from build123d import *

# Parameters (mm, degrees)
ESQUISSE2_R             = 7.5
BOSS_EXTRU_1_DEPTH      = 60
ESQUISSE3_R             = 10
BOSS_EXTRU_2_DEPTH      = 15
ESQUISSE4_R             = 10
BOSS_EXTRU_3_DEPTH      = 15
ESQUISSE5_R             = 7.5
BOSS_EXTRU_4_DEPTH      = 14.25
ENL_V_MAT_EXTRU_1_DEPTH = 16


with BuildPart() as part:
    # Esquisse2 → Boss.-Extru.1 (new body)
    with BuildSketch(Plane.XY):
        Circle(ESQUISSE2_R)
    extrude(amount=BOSS_EXTRU_1_DEPTH)

    # Esquisse3 → Boss.-Extru.2 (add)
    with BuildSketch(Plane.XY.offset(60)):
        with Locations((1.75, 0)):
            Circle(ESQUISSE3_R)
    extrude(amount=BOSS_EXTRU_2_DEPTH)

    # Esquisse4 → Boss.-Extru.3 (add)
    with BuildSketch(Plane.XY.offset(75)):
        with Locations(Location((-1.75, 0, 0), (0, 0, 280.078658108))):
            Circle(ESQUISSE4_R)
    extrude(amount=BOSS_EXTRU_3_DEPTH)

    # Esquisse5 → Boss.-Extru.4 (add)
    with BuildSketch(Plane.XY.offset(90)):
        Circle(ESQUISSE5_R)
    extrude(amount=BOSS_EXTRU_4_DEPTH)

    # Esquisse6 → Enlèv. mat.-Extru.1 (cut)
    with BuildSketch(Plane(origin=(0, 0, 0), x_dir=(-1, 0, 0), z_dir=(0, 0, -1))):
        with BuildLine():
            Line((-2.5, 7.071067812), (-2.5, 5.25))
            Line((-2.5, 5.25), (2.5, 5.25))
            Line((2.5, 5.25), (2.5, 7.071067812))
            ThreePointArc((2.5, 7.071067812), (0, 7.5), (-2.5, 7.071067812))
        make_face()
    extrude(amount=-ENL_V_MAT_EXTRU_1_DEPTH, mode=Mode.SUBTRACT)


solid = part.part
Here's how the part is built. I have some questions about the finished solid (model axes, mm). A direction names the side the tool comes from. Round coordinates to 2 decimals unless told otherwise and drop trailing zeros. Loops run counter-clockwise (first coordinate to the right, second up) from the corner with the lowest first, then second, coordinate; pieces in that order, holes last. Notation, with made-up numbers: (-9, 67) - (32, 67) arc R21 ccw to (32, 106) - close; hole circle Ø3 at (59, -1). An arc over 180 degrees is marked (long way). One line per question, with ' | ' between items. Start each with the question number.
Q1. For faces 1 (the flat face through (2.5, 6, 8)), 2 (the flat face through (-9, 0, 75)), 3 (the flat face through (8.5, 0, 75)), 4 (the cylindrical face through (11.29, 3, 67.4)), which set-ups out of +Z, -Z, +X, -X, +Y, -Y let a thin tool reach every point of the face, with its end or its side?
Q2. I want a section at A-A (y = -4.5). Write out the boundary of the cut face in (x, z).
Q3. Please list where these lines run through material, in increasing order: line 1 (Z direction, x = -3.25, y = -7.5); line 2 (Y direction, x = 0.25, z = 58.5); line 3 (Z direction, x = -10, y = -1.75). Write a range as [from, to].
Q4. I want a section at B-B (x = 1.5). Write out the boundary of the cut face in (y, z).
Q5. I want a section at C-C (z = 32.5). Write out the boundary of the cut face in (x, y), then the cut area to 3 significant figures.
Q6. I want a section at D-D (y = 0). Write out the boundary of the cut face in (x, z).
Q7. Will these pins go through, and if not, where does the flat tip stop? pin 1 (1.5 mm diameter, centred on y = -0.5, z = 40.5, fed in from +X); pin 2 (12 mm diameter, centred on x = -3.5, z = 10.5, fed in from +Y); pin 3 (1.5 mm diameter, centred on y = 6, z = 5.5, fed in from +X); pin 4 (9.5 mm diameter, centred on x = -7.5, y = 1.5, fed in from -Z).
Response values:
1) face 1: -Z, +Y | face 2: -Z, -X | face 3: +Z, +X | face 4: -Z
2) outline: (-10.68, 75) - (-7.18, 75) - (-7.18, 60) - (-6, 60) - (-6, 0) - (6, 0) - (6, 60) - (10.68, 60) - (10.68, 75) - (7.18, 75) - (7.18, 90) - (6, 90) - (6, 104.25) - (-6, 104.25) - (-6, 90) - (-10.68, 90) - close
3) line 1: z = [60, 90] | line 2: y = [-7.5, 7.5] | line 3: z = [75, 90]
4) outline: (-10, 60) - (-7.35, 60) - (-7.35, 0) - (5.25, 0) - (5.25, 16) - (7.35, 16) - (7.35, 60) - (10, 60) - (10, 75) - (9.46, 75) - (9.46, 90) - (7.35, 90) - (7.35, 104.25) - (-7.35, 104.25) - (-7.35, 90) - (-9.46, 90) - (-9.46, 75) - (-10, 75) - close
5) outline: circle Ø15 at (0, 0) | area: 177 mm²
6) outline: (-11.75, 75) - (-8.25, 75) - (-8.25, 60) - (-7.5, 60) - (-7.5, 0) - (7.5, 0) - (7.5, 60) - (11.75, 60) - (11.75, 75) - (8.25, 75) - (8.25, 90) - (7.5, 90) - (7.5, 104.25) - (-7.5, 104.25) - (-7.5, 90) - (-11.75, 90) - close
7) pin 1: stops at x = 7.5 | pin 2: stops at y = 7.42 | pin 3: stops at x = 5.36 | pin 4: stops at z = 0
